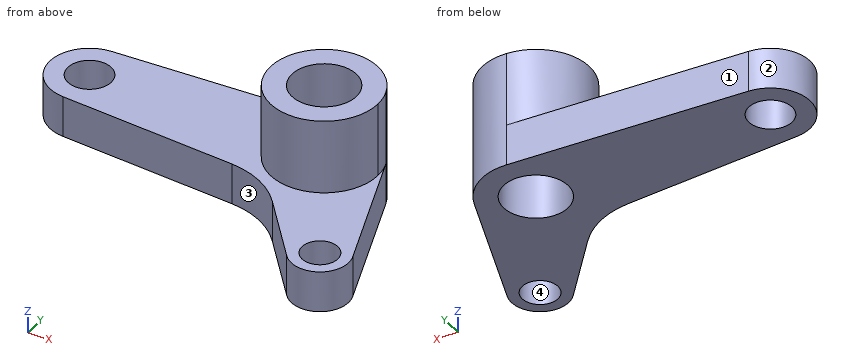
from build123d import *

# Parameters (mm, degrees)
F0_R     = 7.790198
F1_DEPTH = 28
F0_R_2   = 4.327888
F0_R_3   = 5.238237
F2_DEPTH = 10


with BuildPart() as f1:
    # F0 (on Top) → F1 (new body)
    with BuildSketch(Plane.XY):
        with BuildLine():
            ThreePointArc((-0.773386, 12.96061), (-8.903206, -9.450315), (12.983664, 0))
            ThreePointArc((12.983664, 0), (12.787958, 2.245812), (12.206738, 4.423921))
            ThreePointArc((12.206738, 4.423921), (7.134364, 10.847875), (-0.773386, 12.96061))
        make_face()
        Circle(F0_R, mode=Mode.SUBTRACT)
    extrude(amount=F1_DEPTH)

    # F0 (on Top) → F2 (join)
    with BuildSketch(Plane.XY):
        with BuildLine():
            ThreePointArc((12.206738, 4.423921), (12.787958, 2.245812), (12.983664, 0))
            ThreePointArc((12.983664, 0), (-8.903206, -9.450315), (-0.773386, 12.96061))
            Line((-0.773386, 12.96061), (-57.319608, 9.586383))
            ThreePointArc((-57.319608, 9.586383), (-66.351004, 0), (-57.319608, -9.586383))
            Line((-57.319608, -9.586383), (-14.921315, -12.116374))
            ThreePointArc((-14.921315, -12.116374), (-7.136198, -14.208437), (-0.80941, -19.204088))
            Line((-0.80941, -19.204088), (12.0131, -34.442827))
            ThreePointArc((12.0131, -34.442827), (20.773863, -35.981386), (23.821813, -27.625063))
            Line((23.821813, -27.625063), (12.206738, 4.423921))
        make_face()
        with Locations((17.311552, -29.984488)):
            Circle(F0_R_2, mode=Mode.SUBTRACT)
        with Locations((-56.74757, 0)):
            Circle(F0_R_3, mode=Mode.SUBTRACT)
    extrude(amount=F2_DEPTH)


solid = f1.part
Can you work these out from the model? Positions are in its coordinate system, mm. Face numbers are marked on the shaded views. Give positions to 0.01 mm unless a question says otherwise; leave off trailing zeros. Order: outer loops, then holes, each group sorted by start corner. A loop starts at its lowest first (then second) coordinate and runs counter-clockwise, first axis right, second up. Notation, with made-up numbers: M -20.75,-6.75 L 24.25,-6.75 A4 ccw 24.25,-0.75 Z; hole C 68,71 d2. An arc over 180 degrees is marked long. Use a Markdown table: item, result. Add a question column.
Item 1: Suppose I cut it at C-C (z = 21.75). List the corners of the cut face in (x, y) for me.
Item 2: Suppose I cut it at B-B (y = -3.5). List the corners of the cut face in (x, z) for me.
Item 3: Suppose I cut it at A-A (z = 5). List the corners of the cut face in (x, y) for me.
Item 4: If I drill on L1, parallel to Z at x = -41, y = 10; L2, parallel to X at y = -33.5, z = 6.25; L3, parallel to Y at x = 0, z = 20, over which ranges is the centre line in solid material (lowest first)? Write a range as [from, to].
Item 5: Will these pins go through, and if not, where does the flat tip stop? pin 1 (1.5 mm diameter, centred on y = 6, z = 9, fed in from +X); pin 2 (8 mm diameter, centred on x = -52, y = -1, fed in from +Z); pin 3 (5 mm diameter, centred on x = -11.5, z = 3.5, fed in from +Y); pin 4 (8 mm diameter, centred on x = 2.5, y = -17, fed in from -Z).
Item 6: We'd pull the mould along Y, two halves only. Please class the marked faces 1, 2, 3 and 4: +Y half, -Y half, draft (parallel to the pull), parting line (faces both ways), or undercut.
Item 7: Suppose I cut it at D-D (x = -31.5). List the corners of the cut face in (y, z) for me.
Answer sheet:
| question | item | result |
|---|---|---|
| 1 | outline | M -0.77,12.96 A12.98 ccw long 12.98,0 A12.98 ccw 12.21,4.42 A12.98 ccw Z; hole C 0,0 d15.58 |
| 2 | outline | M -65.69,0 L -60.64,0 L -60.64,10 L -65.69,10 Z; M -52.85,0 L -6.96,0 L -6.96,28 L -12.5,28 L -12.5,10 L -52.85,10 Z; M 6.96,0 L 15.08,0 L 15.08,10 L 12.5,10 L 12.5,28 L 6.96,28 Z |
| 3 | outline | M -57.32,-9.59 L -14.92,-12.12 A20 cw -0.81,-19.2 L 12.01,-34.44 A6.92 ccw 23.82,-27.63 L 12.21,4.42 A12.98 ccw -0.77,12.96 L -57.32,9.59 A9.6 ccw Z; hole C -56.75,0 d10.48; hole C 0,0 d15.58; hole C 17.31,-29.98 d8.66 |
| 4 | L1 | z = [0, 10] |
| 4 | L2 | x = [11.22, 14.79], [19.84, 23.28] |
| 4 | L3 | y = [-12.98, -7.79], [7.79, 12.98] |
| 5 | pin 1 | stops at x = 11.87 |
| 5 | pin 2 | stops at z = 10 |
| 5 | pin 3 | stops at y = 12.47 |
| 5 | pin 4 | stops at z = 0 |
| 6 | face 1 | +Y half |
| 6 | face 2 | parting line |
| 6 | face 3 | -Y half |
| 6 | face 4 | undercut |
| 7 | outline | M -11.13,0 L 11.13,0 L 11.13,10 L -11.13,10 Z |
